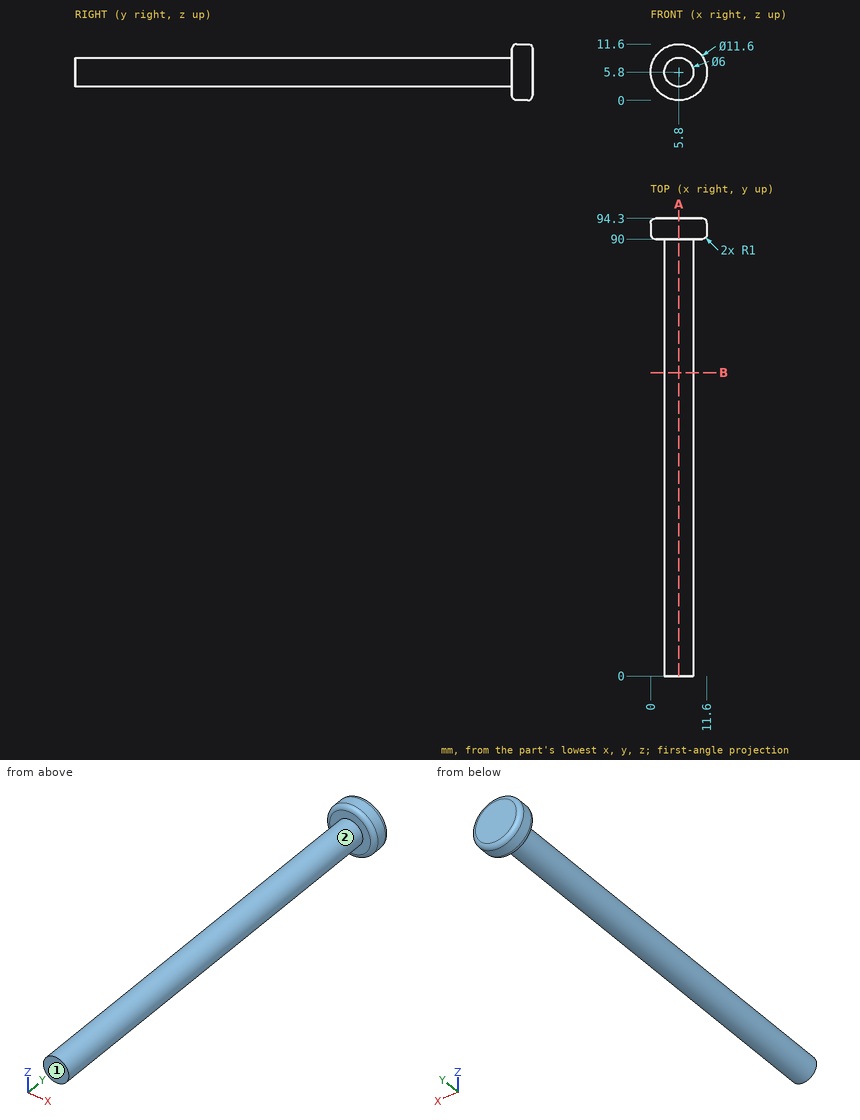
Design review of the part shown in the three views and the two pictorial views. Dimensions are in mm from the part's minimum x, y and z. A direction names the side the tool comes from. Coordinates: 2 decimals unless noted, no trailing zeros. Write each loop counter-clockwise with the first axis right and the second up, starting at its lowest first coordinate (ties: lowest second). Pieces come first, ordered by that corner, then holes.
(1) Add section B-B on y = 62.5. Give the boundary of the cut face in (x, z), then the cut area to 3 significant figures.
(2) Tool access review of the marked faces 1 and 2: name each direction out of +Z, -Z, +X, -X, +Y, -Y from which nothing blocks a thin tool from reaching the whole face with its end or side.
(3) Add section A-A on x = 5.8. Give the boundary of the cut face in (y, z), then the cut area to 3 significant figures.
(4) For pin 1 Ø6 at (x, y) = (3.5, 49.5) entering from -Z; pin 2 Ø3 at (y, z) = (80, 4.5) entering from -X; pin 3 Ø3 at (x, y) = (4, 27.5) entering from +Z, all flat-tipped, find the tip position at first contact; note any pin that passes through.
(5) Wall thickness on probe 1 along Y at (x, z) = (9.75, 6); probe 2 along X at (y, z) = (39, 6); probe 3 along Y at (x, z) = (1, 8.5): over which ranges is each line inside the solid? List them lowest first.
Answer sheet:
1. outline: circle Ø6 at (5.8, 5.8)
1. area: 28.3 mm2
2. face 1: +Z, -Z, +X, -X, -Y
2. face 2: -Y
3. outline: (0, 2.8) - (90, 2.8) - (90, 1) arc R1 ccw to (91, 0) - (93.3, 0) arc R1 ccw to (94.3, 1) - (94.3, 10.6) arc R1 ccw to (93.3, 11.6) - (91, 11.6) arc R1 ccw to (90, 10.6) - (90, 8.8) - (0, 8.8) - close
3. area: 589 mm2
4. pin 1: stops at z = 2.8
4. pin 2: stops at x = 2.8
4. pin 3: stops at z = 8.78
5. probe 1: y = 90 to 94.3
5. probe 2: x = 2.81 to 8.79
5. probe 3: y = 90.29 to 94.01
